from build123d import *

# Parameters (mm, degrees)
SKETCH1_R           = 25.4
BOSS_EXTRUDE1_DEPTH = 38.1
SKETCH2_W           = 88.9
SKETCH2_H           = 179.4002
CUT_EXTRUDE1_DEPTH  = 19.05


with BuildPart() as part:
    # Sketch1 → Boss-Extrude1 (new body)
    with BuildSketch(Plane(origin=(0, 0, 0), x_dir=(1, 0, 0), z_dir=(0, 1, 0))):
        Polygon((685.8127, 0), (0, 0), (0, -179.4002), (590.5627, -179.4002), (590.5627, -141.2875), (685.8127, -141.2875), align=None)
        with Locations((538.1752, -73.918191)):
            Circle(SKETCH1_R, mode=Mode.SUBTRACT)
    extrude(amount=BOSS_EXTRUDE1_DEPTH)

    # Sketch2 → Cut-Extrude1 (cut)
    with BuildSketch(Plane.XZ):
        with Locations((411.15104079, 89.7001)):
            Rectangle(SKETCH2_W, SKETCH2_H)
    extrude(amount=-CUT_EXTRUDE1_DEPTH, mode=Mode.SUBTRACT)


solid = part.part
Geometry: final body of the model. Coordinates: model frame, mm. A direction names the side the tool comes from. Give positions to 0.01 mm unless a question says otherwise; leave off trailing zeros. Write each loop counter-clockwise with the first axis right and the second up, starting at its lowest first coordinate (ties: lowest second). Pieces come first, ordered by that corner, then holes. Notation, with made-up numbers: (-40, 23) -> (-16, 23) arc R30 ccw to (-16, 49) -> close; hole circle Ø8 at (37, 1.5). An arc over 180 degrees is marked (long way). Answer in a Markdown table with one row per item.
(1) Section query B-B on z = 83. Return loops of the section in (x, y), then the cut area to 3 significant figures.
Answers below:
| item | result |
|---|---|
| outline | (0, 0) -> (366.7, 0) -> (366.7, 19.05) -> (455.6, 19.05) -> (455.6, 0) -> (514.45, 0) -> (514.45, 38.1) -> (0, 38.1) -> close; (561.9, 0) -> (685.81, 0) -> (685.81, 38.1) -> (561.9, 38.1) -> close |
| area | 22,600 mm^2 |
(2) Section query D-D on x = 607. Return loops of the section in (y, z).
Answers below:
| item | result |
|---|---|
| outline | (0, 0) -> (38.1, 0) -> (38.1, 141.29) -> (0, 141.29) -> close |
(3) Pin query (flat end, axial travel): pin 1 (11.5 mm diameter, centred on x = 645, y = 18, fed in from +Z). Return the tip coordinate at first contact, or that it passes through.
Answers below:
| item | result |
|---|---|
| pin 1 | z = 141.29 |
(4) Section query A-A on z = 133.5. Return loops of the section in (x, y), then the cut area to 3 significant figures.
Answers below:
| item | result |
|---|---|
| outline | (0, 0) -> (366.7, 0) -> (366.7, 19.05) -> (455.6, 19.05) -> (455.6, 0) -> (685.81, 0) -> (685.81, 38.1) -> (0, 38.1) -> close |
| area | 24,400 mm^2 |
(5) Set-up query: faces 1 (the flat face through (569, 0, 88)), 2 (the flat face through (411, 19.05, 91)), 3 (the flat face through (638, 19, 141.288)). Return all of +Z, -Z, +X, -X, +Y, -Y with unobstructed straight access to the full face (end or side cutting, diameter ignored); none if empty.
Answers below:
| item | result |
|---|---|
| face 1 | +Z, -Z, +X, -X, -Y |
| face 2 | +Z, -Z, -Y |
| face 3 | +Z, +X, +Y, -Y |
(6) Draft query along X for faces 4 (the flat face through (455.601, 9, 88)), 5 (the flat face through (181, 0, 88)), 6 (the flat face through (366.701, 9, 88)), 7 (the flat face through (685.813, 19, 72)). Return one class per face: +X half, -X half, draft (parallel to the pull), parting line (faces both ways), or undercut.
Answers below:
| item | result |
|---|---|
| face 4 | undercut |
| face 5 | draft |
| face 6 | undercut |
| face 7 | +X half |
(7) Section query C-C on y = 31.5. Return loops of the section in (x, z), then the cut area to 3 significant figures.
Answers below:
| item | result |
|---|---|
| outline | (0, 0) -> (685.81, 0) -> (685.81, 141.29) -> (590.56, 141.29) -> (590.56, 179.4) -> (0, 179.4) -> close; hole circle Ø50.8 at (538.18, 73.92) |
| area | 117,000 mm^2 |
(8) Ray query, line 1 along X through (y, z) = (16.5, 115); line 2 along X through (y, z) = (4, 97); line 3 along X through (y, z) = (5, 80). Return the intervals inside material, ascending. Write a range as [from, to].
Answers below:
| item | result |
|---|---|
| line 1 | [0, 366.7], [455.6, 685.81] |
| line 2 | [0, 366.7], [455.6, 527.57], [548.78, 685.81] |
| line 3 | [0, 366.7], [455.6, 513.51], [562.84, 685.81] |
